from build123d import *

# Parameters (mm, degrees)
ESBO_O1_R                = 5
RESSALTO_EXTRUS_O1_DEPTH = 5
CORTE_EXTRUS_O1_DEPTH    = 4
ESBO_O3_R                = 2
CORTE_EXTRUS_O2_DEPTH    = 9.124038405
RESSALTO_EXTRUS_O2_DEPTH = 5
CHANFRO1_SIZE            = 0.5
FILETE1_R                = 2


with BuildPart() as part:
    # Esboço1 → Ressalto-extrusão1 (new body)
    with BuildSketch(Plane.XY):
        Circle(ESBO_O1_R)
    extrude(amount=RESSALTO_EXTRUS_O1_DEPTH)

    # Esboço2 → Corte-extrusão1 (cut)
    with BuildSketch(Plane.XY.offset(5)):
        Polygon((0, 3.175426481), (-2.75, 1.58771324), (-2.75, -1.58771324), (0, -3.175426481), (2.75, -1.58771324), (2.75, 1.58771324), align=None)
    extrude(amount=-CORTE_EXTRUS_O1_DEPTH, mode=Mode.SUBTRACT)

    # Esboço3 → Corte-extrusão2 (cut, through all)
    with BuildSketch(Plane.XY.offset(1)):
        Circle(ESBO_O3_R)
    extrude(amount=-CORTE_EXTRUS_O2_DEPTH, mode=Mode.SUBTRACT)

    # Esboço4 → Ressalto-extrusão2 (add, through all)
    with BuildSketch(Plane(origin=(0, 0, 0), x_dir=(-1, 0, 0), z_dir=(0, 0, -1))):
        with BuildLine():
            Line((-4.582575695, 2), (-8, 2))
            ThreePointArc((-8, 2), (-10, 1.13e-07), (-8.000000226, -2))
            Line((-8.000000226, -2), (-4.582575695, -2))
            ThreePointArc((-4.582575695, -2), (-5, 0), (-4.582575695, 2))
        make_face()
        with BuildLine():
            Line((2, 4.582575695), (2, 8))
            ThreePointArc((2, 8), (1.13e-07, 10), (-2, 8.000000226))
            Line((-2, 8.000000226), (-2, 4.582575695))
            ThreePointArc((-2, 4.582575695), (0, 5), (2, 4.582575695))
        make_face()
        with BuildLine():
            Line((4.582575695, -2), (8, -2))
            ThreePointArc((8, -2), (10, -1.13e-07), (8.000000226, 2))
            Line((8.000000226, 2), (4.582575695, 2))
            ThreePointArc((4.582575695, 2), (5, 0), (4.582575695, -2))
        make_face()
        with BuildLine():
            Line((-2, -4.582575695), (-2, -8))
            ThreePointArc((-2, -8), (-1.13e-07, -10), (2, -8.000000226))
            Line((2, -8.000000226), (2, -4.582575695))
            ThreePointArc((2, -4.582575695), (0, -5), (-2, -4.582575695))
        make_face()
    extrude(amount=-RESSALTO_EXTRUS_O2_DEPTH)

    # Chanfro1
    chanfro1_edges = [part.edges().sort_by_distance(p)[0] for p in [
        (1.375, 2.38156986, 5),
        (-1.375, 2.38156986, 5),
        (-2.75, 0, 5),
        (-1.375, -2.38156986, 5),
        (1.375, -2.38156986, 5),
        (2.75, 0, 5),
    ]]
    chamfer(chanfro1_edges, length=CHANFRO1_SIZE)

    # Filete1
    filete1_edges = [part.edges().sort_by_distance(p)[0] for p in [
        (4.582575695, 2, 2.5),
        (4.582575695, -2, 2.5),
        (-2, 4.582575695, 2.5),
        (2, 4.582575695, 2.5),
        (-4.582575695, -2, 2.5),
        (-4.582575695, 2, 2.5),
        (2, -4.582575695, 2.5),
        (-2, -4.582575695, 2.5),
    ]]
    fillet(filete1_edges, radius=FILETE1_R)


solid = part.part
Could you check a few things on this model? Use its own coordinates, in mm. A direction names the side the tool comes from. Coordinates: 2 decimals unless noted, no trailing zeros. Loops run counter-clockwise (first coordinate to the right, second up) from the corner with the lowest first, then second, coordinate; pieces in that order, holes last.
1. Imagine slicing it at C-C (x = 0.5). Please give me the cut outline in (y, z), and give its area (3 significant figures).
2. I need wall thicknesses on L1, parallel to Y at x = 0, z = 0.5; L2, parallel to X at y = 2.75, z = 1.9; L3, parallel to Y at x = -1.5, z = 0.65. Which ranges of each line are inside material? Lowest first, please.
3. We'd pull the mould along X, two halves only. Please class faces 5 (the face through (-1.394, -2.37, 2.774)), 6 (the face through (-4.81, -2.23, 2.54)), 7 (the face through (7, 2, 2)), 8 (the face through (2.22, 4.83, 2.54)): released by +X, released by -X, zero draft, split by the parting line, or undercut.
4. For P1, Ø2.5, axis at x = -6.5, z = 3.5, coming from the +Y side; P2, Ø5, axis at x = -5, y = 5.5, coming from the +Z side; P3, Ø2, axis at x = -3.5, z = 1, coming from the +Y side; P4, Ø1.1, axis at y = 6.5, z = 2, coming from the -X side, each with a flat end and sliding along its axis, tell me the tip position at first contact or that it passes through.
5. Imagine slicing it at A-A (y = 0). Please give me the cut outline in (x, z), and give its area (4 significant figures).
6. Imagine slicing it at D-D (y = -7). Please give me the cut outline in (x, z), and give its area (3 significant figures).
7. For faces 1 (the face through (-1.48, 2.61, 4.75)), 2 (the face through (-7, 2, 2)), 3 (the face through (3.54, 3.53, 2.46)), 4 (the face through (2, -7, 2)), which set-ups out of +Z, -Z, +X, -X, +Y, -Y let a thin tool reach every point of the face, with its end or its side?
Computed values:
1. outline: (-9.94, 0) - (-1.94, 0) - (-1.94, 1) - (-2.89, 1) - (-2.89, 4.5) - (-3.46, 5) - (-9.94, 5) - close; (1.94, 0) - (9.94, 0) - (9.94, 5) - (3.46, 5) - (2.89, 4.5) - (2.89, 1) - (1.94, 1) - close
1. area: 72.1 mm2
2. L1: y = -10 to -2, 2 to 10
2. L2: x = -4.18 to -0.74, 0.74 to 4.18
2. L3: y = -9.32 to -1.32, 1.32 to 9.32
3. face 5: undercut
3. face 6: released by -X
3. face 7: zero draft
3. face 8: released by +X
4. P1: stops at y = 2.06
4. P2: stops at z = 5
4. P3: stops at y = 4.42
4. P4: stops at x = -2
5. outline: (-10, 0) - (-2, 0) - (-2, 1) - (-2.75, 1) - (-2.75, 4.5) - (-3.25, 5) - (-10, 5) - close; (2, 0) - (10, 0) - (10, 5) - (3.25, 5) - (2.75, 4.5) - (2.75, 1) - (2, 1) - close
5. area: 73.75 mm2
6. outline: (-2, 0) - (2, 0) - (2, 5) - (-2, 5) - close
6. area: 20.0 mm2
7. face 1: +Z
7. face 2: +Z, -Z, -X, +Y
7. face 3: +Z, -Z, +X, +Y
7. face 4: +Z, -Z, +X, -Y
